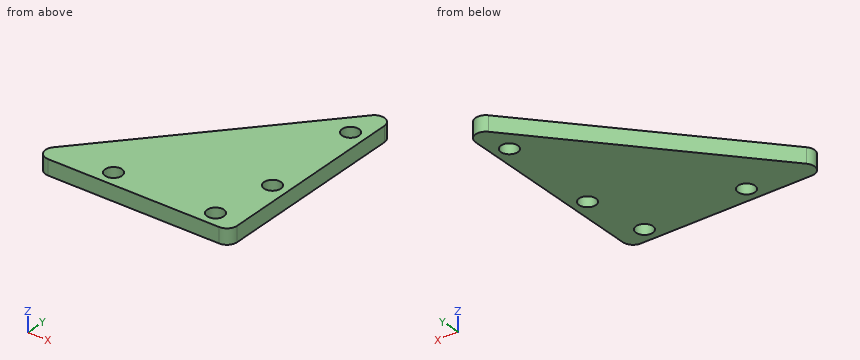
from build123d import *

# Parameters (mm, degrees)
EXTRUDE_1_DEPTH     = 3
SKETCH_2_R          = 1.65
CUT_EXTRUDE_1_DEPTH = 3
SKETCH_3_R          = 1.65
CUT_EXTRUDE_2_DEPTH = 3
FILLET_1_R          = 2


with BuildPart() as part:
    # 草图1 → 凸台-拉伸1 (new body)
    with BuildSketch(Plane.XY):
        Polygon((0, 0), (-40, 0), (0, 45), align=None)
    extrude(amount=EXTRUDE_1_DEPTH)

    # 草图2 → 切除-拉伸1 (cut)
    with BuildSketch(Plane.XY.offset(3)):
        with Locations((-5, 3)):
            Circle(SKETCH_2_R)
        with Locations((-25, 3)):
            Circle(SKETCH_2_R)
    extrude(amount=-CUT_EXTRUDE_1_DEPTH, mode=Mode.SUBTRACT)

    # 草图3 → 切除-拉伸2 (cut)
    with BuildSketch(Plane.XY.offset(3)):
        with Locations((-3, 15)):
            Circle(SKETCH_3_R)
        with Locations((-3, 35)):
            Circle(SKETCH_3_R)
    extrude(amount=-CUT_EXTRUDE_2_DEPTH, mode=Mode.SUBTRACT)

    # 圆角1
    fillet_1_edges = [part.edges().sort_by_distance(p)[0] for p in [
        (0, 0, 1.5),
        (-40, 0, 1.5),
        (0, 45, 1.5),
    ]]
    fillet(fillet_1_edges, radius=FILLET_1_R)


solid = part.part
The listing builds one solid part. Answer for the finished solid, in the listing's coordinates (mm). Give positions to 0.01 mm unless a question says otherwise; leave off trailing zeros. Write each loop counter-clockwise with the first axis right and the second up, starting at its lowest first coordinate (ties: lowest second). Pieces come first, ordered by that corner, then holes.
Item 1: Section C-C, the plane y = 15 is taken. Write down the section's boundary in (x, z), plus the area to 3 significant figures.
Item 2: Section B-B, the plane z = 1.95 is taken. Write down the section's boundary in (x, y), plus the area to 3 significant figures.
Item 3: Flat-ended cylindrical pins translate along their axes: P1, Ø4.5, axis at x = -3, y = 15, coming from the +Z side; P2, Ø1.5, axis at y = 13.5, z = 2, coming from the -X side; P3, Ø1, axis at y = 17.5, z = 1, coming from the -X side; P4, Ø3, axis at x = -3, y = 35, coming from the +Z side. Find the tip coordinate at first contact, or state that the pin passes through.
Item 4: Section A-A, the plane x = -25.5 is taken. Write down the section's boundary in (y, z), plus the area to 3 significant figures.
Item 5: Section D-D, the plane x = -14 is taken. Write down the section's boundary in (y, z), plus the area to 4 significant figures.
Item 6: Find the intervals of material crossed by line 1 along Y through (x, z) = (-3, 1.85); line 2 along Y through (x, z) = (-25, 1.75) (3 decimals); line 3 along Y through (x, z) = (-24, 1.55), in increasing order.
Completed:
1. outline: (-26.67, 0) - (-4.65, 0) - (-4.65, 3) - (-26.67, 3) - close; (-1.35, 0) - (0, 0) - (0, 3) - (-1.35, 3) - close
1. area: 70.1 mm2
2. outline: (-37.04, 3.33) arc R2 ccw to (-35.55, 0) - (-2, 0) arc R2 ccw to (0, 2) - (0, 39.74) arc R2 ccw to (-3.49, 41.07) - close; hole circle Ø3.3 at (-25, 3); hole circle Ø3.3 at (-5, 3); hole circle Ø3.3 at (-3, 15); hole circle Ø3.3 at (-3, 35)
2. area: 855 mm2
3. P1: stops at z = 3
3. P2: stops at x = -28.67
3. P3: stops at x = -24.89
3. P4: passes through
4. outline: (0, 0) - (1.43, 0) - (1.43, 3) - (0, 3) - close; (4.57, 0) - (16.31, 0) - (16.31, 3) - (4.57, 3) - close
4. area: 39.5 mm2
5. outline: (0, 0) - (29.25, 0) - (29.25, 3) - (0, 3) - close
5. area: 87.75 mm2
6. line 1: y = 0 to 13.35, 16.65 to 33.35, 36.65 to 41.47
6. line 2: y = 0 to 1.35, 4.65 to 16.875
6. line 3: y = 0 to 1.69, 4.31 to 18
